Autodesk Inventor part; units mm, degrees
ref_plane "YZ Plane" through (0, 0, 0) normal (1, 0, 0) x (0, 1, 0)
ref_plane "XZ Plane" through (0, 0, 0) normal (0, 1, 0) x (-1, 0, 0)
ref_plane "XY Plane" through (0, 0, 0) normal (0, 0, 1) x (1, 0, 0)
sketch "Sketch1" plane through (0, 0, 0) normal (0, 1, 0) x (-1, 0, 0)
  circle A0 centre (0, 0) radius 20 construction
  circle A1 centre (0, 20) radius 20
  circle A2 centre (0, 0) radius 20 construction
  circle A3 centre (-17.3205, -10) radius 20
  circle A4 centre (0, 0) radius 20 construction
  circle A5 centre (17.3205, -10) radius 20
  dimension "d0" = 40
  dimension "d1" = 40
  dimension "d4" = 360
extrude "Extrusion1" add sketch "Sketch1" along normal blind 20
fillet "Fillet1" radius 10 1 edges at (0, 10, -20)
fillet "Fillet2" radius 10 1 edges at (-17.3205, 10, 10)
fillet "Fillet3" radius 10 1 edges at (17.3205, 10, 10)
sketch "Sketch2" plane through (0, 0, 0) normal (0, 1, 0) x (-1, 0, 0)
  circle A0 centre (0, 0) radius 10
  dimension "d11" = 20
extrude "Extrusion2" add sketch "Sketch2" against normal blind 10
sketch "Sketch3" plane through (0, 0, 0) normal (0, 0, 1) x (1, 0, 0)
  circle A0 centre (0, -5) radius 2
  line L0 (-10, -10) -> (10, -10)
  point P0 (0, 0)
  dimension "d14" = 4
  dimension "d15" = 5
extrude "Extrusion3" cut sketch "Sketch3" along normal through all both and the other way through all
sketch "Sketch4" plane through (0, -10, 0) normal (0, -1, 0) x (1, 0, 0)
  circle A0 centre (0, 0) radius 3.25
  dimension "d18" = 6.5
extrude "Extrusion4" cut sketch "Sketch4" against normal blind 15
sketch "Sketch6" plane through (0, 20, 0) normal (0, 1, 0) x (1, 0, 0)
  circle A0 centre (0, 0) radius 20
  dimension "d26" = 40
extrude "Extrusion5" add sketch "Sketch6" along normal blind 20
sketch "Sketch7" plane through (0, 40, 0) normal (0, 1, 0) x (1, 0, 0)
  circle A0 centre (0, 0) radius 20 construction
  circle A1 centre (0, 20) radius 20
  circle A2 centre (0, 0) radius 20 construction
  circle A3 centre (-17.3205, -10) radius 20
  circle A4 centre (0, 0) radius 20 construction
  circle A5 centre (17.3205, -10) radius 20
  dimension "d31" = 40
  dimension "d32" = 40
  dimension "d33" = 360
extrude "Extrusion6" add sketch "Sketch7" along normal blind 20
fillet "Fillet4" radius 10 3 edges at (17.3205, 50, -10) (-17.3205, 50, -10) (0, 50, 20)
equation "\"d1\" = d0"
equation "\"d32\" = d31"
properties part number "field-mover"
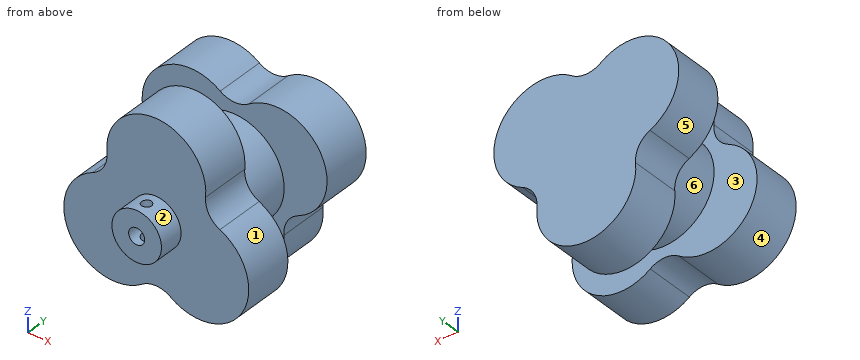
Geometry check sheet. Reference: the model listing, model coordinates, mm. Face numbers are marked on the shaded views. A direction names the side the tool comes from. Round coordinates to 2 decimals unless told otherwise and drop trailing zeros. Write each loop counter-clockwise with the first axis right and the second up, starting at its lowest first coordinate (ties: lowest second). Pieces come first, ordered by that corner, then holes.
Item 1: Material ranges on line 1 along Y through (x, z) = (0, 6.5); line 2 along Y through (x, z) = (6.5, 22); line 3 along Y through (x, z) = (25.5, -20), recorded low to high.
Determined:
line 1: y = -10 to -7, -3 to 60
line 2: y = 0 to 20, 40 to 60
line 3: y = 0 to 20
Item 2: Mould release check, pull along X, two halves, no side actions. Record for the marked faces 1, 2 and 3: +X half, -X half, draft (parallel to the pull), parting line (faces both ways), or undercut.
Determined:
face 1: undercut
face 2: parting line
face 3: draft
Item 3: Go/stop test with flat-tipped pins: pin 1 Ø4 at (x, y) = (10.5, 41.5) entering from -Z; pin 2 Ø5 at (x, y) = (0, -5) entering from +Z; pin 3 Ø6 at (y, z) = (15, -2) entering from +X. Record where each tip stops, or that it passes through.
Determined:
pin 1: stops at z = -38.1
pin 2: stops at z = 10
pin 3: stops at x = 36.69
Item 4: Section check B-B (z = 0). Record the boundary of the cut face in (x, y).
Determined:
outline: (-34.64, 0) - (-10, 0) - (-10, -10) - (-3.25, -10) - (-3.25, 5) - (3.25, 5) - (3.25, -10) - (10, -10) - (10, 0) - (34.64, 0) - (34.64, 20) - (20, 20) - (20, 40) - (34.64, 40) - (34.64, 60) - (-34.64, 60) - (-34.64, 40) - (-20, 40) - (-20, 20) - (-34.64, 20) - close
Item 5: Section check A-A (y = -5). Record the boundary of the cut face in (x, z), plus the area to 3 significant figures.
Determined:
outline: (-2, -9.8) - (-2, -2.56) arc R3.25 cw to (-2, 2.56) - (-2, 9.8) arc R10 ccw to start; (2, -9.8) arc R10 ccw to (2, 9.8) - (2, 2.56) arc R3.25 cw to (2, -2.56) - close
area: 226 mm2
Item 6: Access from +Z, -Z, +X, -X, +Y, -Y to the whole of each face (thin tool, end or side, straight path). Record for the marked faces 4, 5 and 6.
Determined:
face 4: -Y
face 5: +Y
face 6: none
Item 7: Section check D-D (x = 0). Give the number of separate pieces and of enclosed holes in the cut face, plus the area to 3 significant figures.
Determined:
separate pieces: 3
enclosed holes: 0
area: 3,430 mm2
Item 8: Section check C-C (x = -18.5). Record the boundary of the cut face in (y, z).
Determined:
outline: (0, -29.97) - (20, -29.97) - (20, -7.6) - (40, -7.6) - (40, -27.6) - (60, -27.6) - (60, 29.97) - (40, 29.97) - (40, 7.6) - (20, 7.6) - (20, 27.6) - (0, 27.6) - close
